CAD build for the part. Positions are in the model's coordinates, mm. A direction names the side the tool comes from. Round coordinates to 2 decimals unless told otherwise and drop trailing zeros. Order: outer loops, then holes, each group sorted by start corner. A loop starts at its lowest first (then second) coordinate and runs counter-clockwise, first axis right, second up. Notation, with made-up numbers: M 24,27.5 L 83,27.5 A19 cw 83,35.5 Z; hole C 51,33.25 d2. An arc over 180 degrees is marked long. Answer as a JSON object with one key per item and string values. Group by question number.
```python
from build123d import *

# Parameters (mm, degrees)
F0_W      = 2.8
F0_H      = 22
F1_DEPTH  = 11
F2_R      = 2
F4_DEPTH  = 19
F5_R      = 3
F6_DEPTH  = 15
F8_DEPTH  = 11
F9_R      = 1
F10_W     = 20
F10_H     = 20
F11_DEPTH = 38.2
F12_R     = 1
F5_R_2    = 6.5
F13_DEPTH = 2.2


with BuildPart() as f1:
    # F0 (on Top) → F1 (new body, symmetric)
    with BuildSketch(Plane.XY):
        with Locations((1.4, 0)):
            Rectangle(F0_W, F0_H)
    extrude(amount=F1_DEPTH, both=True)

    # F2
    f2_edges = [f1.edges().sort_by_distance(p)[0] for p in [
        (1.4, -11, 11),
        (1.4, 11, 11),
        (1.4, -11, -11),
        (1.4, 11, -11),
    ]]
    fillet(f2_edges, radius=F2_R)

    # F3 (on face) → F4 (join)
    with BuildSketch(Plane.YZ.offset(2.8)):
        with BuildLine():
            ThreePointArc((0, -11), (7.7781745931, -7.7781745931), (11, 0))
            ThreePointArc((11, 0), (7.7781745931, 7.7781745931), (0, 11))
            ThreePointArc((0, 11), (-7.7781745931, 7.7781745931), (-11, 0))
            ThreePointArc((-11, 0), (-7.7781745931, -7.7781745931), (0, -11))
        make_face()
    extrude(amount=F4_DEPTH)

    # F5 (on face) → F6 (join)
    with BuildSketch(Plane.YZ.offset(21.8)):
        Circle(F5_R)
    extrude(amount=F6_DEPTH)

    # F7 (on face) → F8 (cut)
    with BuildSketch(Plane.YZ.offset(36.8)):
        with BuildLine():
            ThreePointArc((2.5980762114, 1.5), (0, 3), (-2.5980762114, 1.5))
            Line((-2.5980762114, 1.5), (2.5980762114, 1.5))
        make_face()
    extrude(amount=-F8_DEPTH, mode=Mode.SUBTRACT)

    # F9
    f9_edges = [f1.edges().sort_by_distance(p)[0] for p in [
        (25.8, 0, 1.5),
    ]]
    fillet(f9_edges, radius=F9_R)

    # F10 (on face) → F11 (join)
    with BuildSketch(Plane(origin=(0, 0, 0), x_dir=(0, -1, 0), z_dir=(-1, 0, 0))):
        Rectangle(F10_W, F10_H)
    extrude(amount=F11_DEPTH)

    # F12
    f12_edges = [f1.edges().sort_by_distance(p)[0] for p in [
        (-19.1, -10, 10),
        (-19.1, 10, 10),
        (-19.1, -10, -10),
        (-19.1, 10, -10),
    ]]
    fillet(f12_edges, radius=F12_R)

    # F5 (on face) → F13 (join)
    with BuildSketch(Plane.YZ.offset(21.8)):
        Circle(F5_R_2)
        Circle(F5_R, mode=Mode.SUBTRACT)
    extrude(amount=F13_DEPTH)


solid = f1.part
```
Item 1: 3-axis set-ups, long thin cutter, end or side, ignore diameter. For faces 1 (the face through (2.8, -8, -8)), 2 (the face through (22.885, -5.158, -3.955)), 3 (the face through (2.8, -8, 9)): which of +Z, -Z, +X, -X, +Y, -Y reach the whole face in a straight line?
Item 2: Cut at D-D, the plane y = -5. Give the cut face in (x, z), and give its area (3 significant figures).
Item 3: Cut at C-C, the plane y = 8.25. Give the cut face in (x, z), and give its area (3 significant figures).
Item 4: Cut at A-A, the plane x = -32. Give the cut face in (y, z), and give its area (3 significant figures).
Item 5: Drill centre lines: line 1 (X direction, y = -4.5, z = 2.5); line 2 (Y direction, x = -16, z = 3). Where is each one in solid material? Low to high. Write a range as [from, to].
Item 6: Flat gauge pins, fed straight in: pin 1 Ø1 at (x, y) = (4, -3.5) entering from +Z; pin 2 Ø4 at (x, y) = (33, 0.5) entering from +Z; pin 3 Ø4 at (x, y) = (-6, -8) entering from -Z. Where does each tip first touch, or does it go through?
Item 7: Cut at B-B, the plane z = 4. Give the cut face in (x, y).
Response values:
{
 "1": {"face 1": "-Z, +X, -Y", "face 2": "+X", "face 3": "+Z, +X, -Y"},
 "2": {"outline": "M -38.2,-10 L 0,-10 L 0,-11 L 2.8,-11 L 2.8,-9.8 L 21.8,-9.8 L 21.8,-4.15 L 24,-4.15 L 24,4.15 L 21.8,4.15 L 21.8,9.8 L 2.8,9.8 L 2.8,11 L 0,11 L 0,10 L -38.2,10 Z", "area": "1,220 mm^2"},
 "3": {"outline": "M -38.2,-10 L 0,-10 L 0,-11 L 2.8,-11 L 2.8,-7.28 L 21.8,-7.28 L 21.8,7.28 L 2.8,7.28 L 2.8,11 L 0,11 L 0,10 L -38.2,10 Z", "area": "1,100 mm^2"},
 "4": {"outline": "M -10,-9 A1 ccw -9,-10 L 9,-10 A1 ccw 10,-9 L 10,9 A1 ccw 9,10 L -9,10 A1 ccw -10,9 Z", "area": "399 mm^2"},
 "5": {"line 1": "[-38.2, 24]", "line 2": "[-10, 10]"},
 "6": {"pin 1": "z = 10.58", "pin 2": "z = 1.5", "pin 3": "z = -10"},
 "7": {"outline": "M -38.2,-10 L 0,-10 L 0,-11 L 2.8,-11 L 2.8,-10.25 L 21.8,-10.25 L 21.8,-5.12 L 24,-5.12 L 24,5.12 L 21.8,5.12 L 21.8,10.25 L 2.8,10.25 L 2.8,11 L 0,11 L 0,10 L -38.2,10 Z"}
}
